```python
from build123d import *

# Parameters (mm, degrees)
F1_DEPTH = 18
F2_T     = -2.2
F4_DEPTH = 18
F3_W     = 13.6
F3_H     = 14.9906637612
F5_DEPTH = 8.9
F6_DEPTH = 2.8


# Not quite as in the source:
# - a feature of the source that left no trace in its solid (it failed there, or was rolled back) is left out


with BuildPart() as f1:
    # F0 (on Right) → F1 (new body)
    with BuildSketch(Plane.YZ):
        Polygon((0, 15), (0, 0), (15, 0), align=None)
    extrude(amount=F1_DEPTH)

    # F2
    f2_openings = [f1.faces().sort_by_distance(p)[0] for p in [
        (9, 7.5, 7.5),
    ]]
    offset(amount=F2_T, openings=f2_openings)

    # F0 (on Right) → F4 (join)
    with BuildSketch(Plane.YZ):
        Polygon((15, 0), (0, 0), (0, 15), (2.8284271247, 15), (-2, 19.8284271247), (-2, -2), (19.8284271247, -2), (15, 2.8284271247), align=None)
        Polygon((0, 15), (15, 0), (15, 2.8284271247), (2.8284271247, 15), align=None)
    extrude(amount=F4_DEPTH)

    # F3 (on face) → F5 (cut)
    with BuildSketch(Plane(origin=(0, 7.5, 7.5), x_dir=(1, 0, 0), z_dir=(0, 0.7071067812, 0.7071067812))):
        with Locations((9, 0)):
            Rectangle(F3_W, F3_H)
    extrude(amount=F5_DEPTH, mode=Mode.SUBTRACT)

    # F6 (add): a face of the model
    f6_faces = [f1.faces().sort_by_distance(p)[0] for p in [
        (9, 19.5757454612, -1.7473183365),
    ]]
    extrude(f6_faces, amount=F6_DEPTH)


solid = f1.part
```
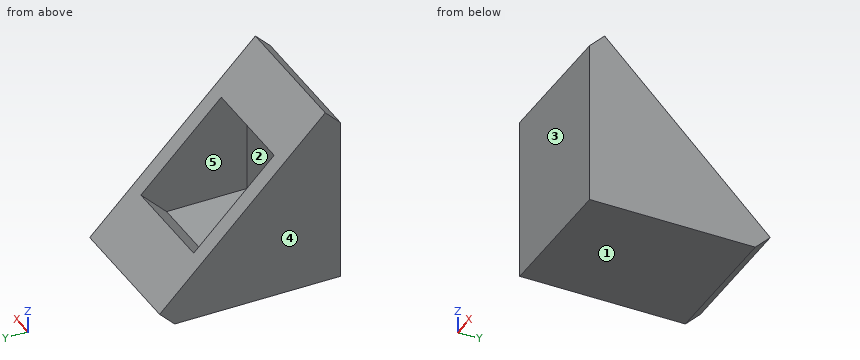
Can you work these out from the model? Positions are in its coordinate system, mm. Face numbers are marked on the shaded views. A direction names the side the tool comes from. Give positions to 0.01 mm unless a question says otherwise; leave off trailing zeros. Write each loop counter-clockwise with the first axis right and the second up, starting at its lowest first coordinate (ties: lowest second). Pieces come first, ordered by that corner, then holes. Notation, with made-up numbers: (73, 88.5) - (132, 88.5) arc R23 cw to (132, 102.5) - close; hole circle Ø6 at (72.25, 34). An arc over 180 degrees is marked (long way). Write item = value, one per line. Start each with the question number.
1. Imagine slicing it at D-D (z = 15.25). Please give me the cut outline in (x, y).
2. Imagine slicing it at A-A (z = 4.25). Please give me the cut outline in (x, y).
3. On a 3-axis mill with a long thin cutter (end or side, diameter ignored), from which of +Z, -Z, +X, -X, +Y, -Y can I reach the whole of each face in a straight line? I mean the marked faces 4 and 5. Say none if no direction works.
4. Imagine slicing it at C-C (x = 5.5). Please give me the cut outline in (y, z), and give its area (3 significant figures).
5. For pin 1 (7 mm diameter, centred on y = 10.5, z = 11.5, fed in from -X); pin 2 (5.5 mm diameter, centred on x = 10.5, z = 8, fed in from +Y); pin 3 (3 mm diameter, centred on x = 10.5, z = 2, fed in from +Y); pin 4 (3 mm diameter, centred on x = 12, y = 9.5, fed in from +Z), each with a flat end and sliding along its axis, tell me the tip position at first contact or that it passes through.
6. Imagine slicing it at B-B (y = 2.75). Please give me the cut outline in (x, z).
7. Please list where these lines run through material, in increasing order: line 1 (X direction, y = 2.5, z = 12.75); line 2 (Z direction, x = 11.75, y = 10).
8. Thinking about a two-plate mould opening in Y: for the marked faces 1, 2 and 3, which applies, released by +Y, released by -Y, zero draft, split by the parting line, or undercut?
Worked answers:
q1.outline = (0, -2) - (18, -2) - (18, 6.54) - (15.8, 6.54) - (15.8, 4.65) - (2.2, 4.65) - (2.2, 6.54) - (0, 6.54) - close
q2.outline = (0, -2) - (18, -2) - (18, 17.54) - (0, 17.54) - close; hole (2.2, 2.2) - (15.8, 2.2) - (15.8, 14.85) - (2.2, 14.85) - close
q3.face_4 = +Z, -Z, -X, +Y, -Y
q3.face_5 = none
q4.outline = (-2, -2) - (19.83, -2) - (21.81, -0.02) - (16.19, 5.59) - (12.8, 2.2) - (2.2, 2.2) - (2.2, 12.8) - (5.59, 16.19) - (-0.02, 21.81) - (-2, 19.83) - close
q4.area = 197 mm2
q5.pin_1 = 0
q5.pin_2 = 16.54
q5.pin_3 = 21.29
q5.pin_4 = 2.2
q6.outline = (0, -2) - (18, -2) - (18, 19.04) - (0, 19.04) - close; hole (2.2, 2.2) - (15.8, 2.2) - (15.8, 13.35) - (2.2, 13.35) - close
q7.line_1 = 0 to 2.2, 15.8 to 18
q7.line_2 = -2 to 2.2
q8.face_1 = zero draft
q8.face_2 = undercut
q8.face_3 = released by -Y
